```python
from build123d import *

# Parameters (mm, degrees)
SKETCH_1_R          = 7.5
EXTRUDE_1_DEPTH     = 2
SKETCH_2_R          = 9.5
EXTRUDE_2_DEPTH     = 7
EXTRUDE_2_TAPER     = 30
SKETCH_4_R          = 3.8
CUT_EXTRUDE_1_DEPTH = 3
CUT_EXTRUDE_2_DEPTH = 17.170961802


with BuildPart() as part:
    # 草图1 → 凸台-拉伸1 (new body)
    with BuildSketch(Plane(origin=(0, 0, 0), x_dir=(1, 0, 0), z_dir=(0, 1, 0))):
        with Locations(Location((0, 0, 0), (0, 0, 270))):
            Circle(SKETCH_1_R)
    extrude(amount=EXTRUDE_1_DEPTH)

    # 草图2 → 凸台-拉伸2 (add)
    with BuildSketch(Plane(origin=(0, 2, 0), x_dir=(1, 0, 0), z_dir=(0, 1, 0))):
        Circle(SKETCH_2_R)
    extrude(amount=EXTRUDE_2_DEPTH, taper=EXTRUDE_2_TAPER)

    # 草图4 → 切除-拉伸1 (cut)
    with BuildSketch(Plane(origin=(0, 9, 0), x_dir=(1, 0, 0), z_dir=(0, 1, 0))):
        with Locations(Location((0, 0, 0), (0, 0, 270))):
            Circle(SKETCH_4_R)
    extrude(amount=-CUT_EXTRUDE_1_DEPTH, mode=Mode.SUBTRACT)

    # 草图5 → 切除-拉伸2 (cut, through all)
    with BuildSketch(Plane(origin=(0, 0, 0), x_dir=(-1, 0, 0), z_dir=(0, -1, 0))):
        with BuildLine():
            Line((1.3, -2.3), (-11.887634873, -2.3))
            Line((-11.887634873, -2.3), (-11.887634873, 2.3))
            Line((-11.887634873, 2.3), (1.3, 2.3))
            ThreePointArc((1.3, 2.3), (2.714213562, 1.714213562), (3.3, 0.3))
            Line((3.3, 0.3), (3.3, -0.3))
            ThreePointArc((3.3, -0.3), (2.714213562, -1.714213562), (1.3, -2.3))
        make_face()
    extrude(amount=-CUT_EXTRUDE_2_DEPTH, mode=Mode.SUBTRACT)


solid = part.part
```
Build history of the part. All positions in model axes, mm. A direction names the side the tool comes from. Give positions to 0.01 mm unless a question says otherwise; leave off trailing zeros. Loops run counter-clockwise (first coordinate to the right, second up) from the corner with the lowest first, then second, coordinate; pieces in that order, holes last. Notation, with made-up numbers: (5, 56) -> (55, 56) arc R32 ccw to (55, 94) -> close; hole circle Ø1 at (-7, 67). An arc over 180 degrees is marked (long way). One line per question, with ' | ' between items.
Q1. Pull direction X, two halves, no side cores. Call faces 1 (the cylindrical face through (-2.7, 2.96, -1.73)), 2 (the flat face through (-1, 6, -3)), 3 (the conical face through (-5.65, 8.66, -0.23)): pulls with the +X half, pulls with the -X half, needs draft (parallel to the pull), parting line crosses it, or undercut.
Filled sheet:
face 1: pulls with the +X half | face 2: undercut | face 3: parting line crosses it
Q2. Cut at A-A, the plane x = 0. Write the cut outline in (y, z).
Filled sheet:
outline: (0, -7.5) -> (2, -7.5) -> (2, -9.5) -> (9, -5.46) -> (9, -3.8) -> (6, -3.8) -> (6, -2.3) -> (0, -2.3) -> close; (0, 2.3) -> (6, 2.3) -> (6, 3.8) -> (9, 3.8) -> (9, 5.46) -> (2, 9.5) -> (2, 7.5) -> (0, 7.5) -> close
Q3. Cut at D-D, the plane y = 5.75. Write the cut outline in (x, z) (3 decimals), plus the area to 3 significant figures.
Filled sheet:
outline: (-3.3, -0.3) -> (-3.3, 0.3) arc R2 cw to (-1.3, 2.3) -> (6.965, 2.3) arc R7.335 ccw (long way) to (6.965, -2.3) -> (-1.3, -2.3) arc R2 cw to start | area: 122 mm²
Q4. Drill centre lines: line 1 along Z through (x, y) = (2.25, 6.25); line 2 along Z through (x, y) = (-3, 2.25); line 3 along Y through (x, z) = (3, 4.75). Where is each one in solid material? Low to high. Write a range as [from, to].
Filled sheet:
line 1: z = [-6.68, -3.06], [3.06, 6.68] | line 2: z = [-8.86, -1.35], [1.35, 8.86] | line 3: y = [0, 8.72]
Q5. Tool access for faces 4 (the flat face through (4, 3, -2.3)), 5 (the cylindrical face through (-3.8, 7.5, -0.1)), 6 (the flat face through (-6, 2, -5)): list every direction of +Z, -Z, +X, -X, +Y, -Y with a clear straight run to the whole face (end or side of a thin tool).
Filled sheet:
face 4: +X, +Y, -Y | face 5: +Y | face 6: -Y
Q6. Drop flat-ended pins along their axis: pin 1 (0.5 mm diameter, centred on y = 4, z = 0, fed in from +X); pin 2 (2.5 mm diameter, centred on x = 5, y = 6.5, fed in from -Z); pin 3 (5 mm diameter, centred on x = -2.5, y = 5.5, fed in from -Z). Give the stop position or say it passes through.
Filled sheet:
pin 1: stops at x = -3.3 | pin 2: stops at z = -6.16 | pin 3: stops at z = -8.68
Q7. Cut at C-C, the plane y = 1.75. Write the cut outline in (x, z), plus the area to 3 significant figures.
Filled sheet:
outline: (-3.3, -0.3) -> (-3.3, 0.3) arc R2 cw to (-1.3, 2.3) -> (7.14, 2.3) arc R7.5 ccw (long way) to (7.14, -2.3) -> (-1.3, -2.3) arc R2 cw to start | area: 129 mm²
Q8. Cut at B-B, the plane z = 0. Write the cut outline in (x, y), plus the area to 3 significant figures.
Filled sheet:
outline: (-9.5, 2) -> (-7.5, 2) -> (-7.5, 0) -> (-3.3, 0) -> (-3.3, 6) -> (-3.8, 6) -> (-3.8, 9) -> (-5.46, 9) -> close | area: 36.2 mm²
